```python
from build123d import *

# Parameters (mm, degrees)
F1_DEPTH = 18
F2_R     = 7.5
F3_DEPTH = 25
F4_R     = 1
F5_SIZE  = 1


with BuildPart() as f1:
    # F0 (on Top) → F1 (new body)
    with BuildSketch(Plane.XY):
        with BuildLine():
            Line((-67.585714, 12.773849), (-90.89085, 17.178571))
            ThreePointArc((-90.89085, 17.178571), (-92.5, 0), (-90.89085, -17.178571))
            Line((-90.89085, -17.178571), (-67.585714, -12.773849))
            ThreePointArc((-67.585714, -12.773849), (-57, 0), (-67.585714, 12.773849))
        make_face()
    extrude(amount=F1_DEPTH)

    # F2 (on face) → F3 (join)
    with BuildSketch(Plane.XY.offset(18)):
        with Locations((-70, 0)):
            Circle(F2_R)
    extrude(amount=F3_DEPTH)

    # F4
    f4_edges = [f1.edges().sort_by_distance(p)[0] for p in [
        (-77.5, 0, 18),
        (-79.238282, 14.97621, 18),
    ]]
    fillet(f4_edges, radius=F4_R)

    # F5
    f5_edges = [f1.edges().sort_by_distance(p)[0] for p in [
        (-77.5, 0, 43),
    ]]
    chamfer(f5_edges, length=F5_SIZE)


solid = f1.part
```
Here's how the part is built. I have some questions about the finished solid (model axes, mm). A direction names the side the tool comes from. Coordinates: 2 decimals unless noted, no trailing zeros. Order: outer loops, then holes, each group sorted by start corner. A loop starts at its lowest first (then second) coordinate and runs counter-clockwise, first axis right, second up. Notation, with made-up numbers: (76.5, 20) - (89.5, 20) arc R14 cw to (89.5, 26) - close; hole circle Ø1 at (52.25, 40). An arc over 180 degrees is marked (long way). One line per question, with ' | ' between items.
(1) Suppose I cut it at C-C on z = 4.5. List the corners of the cut face in (x, y) for me, and give its area (3 significant figures).
Report:
outline: (-90.89, -17.18) - (-67.59, -12.77) arc R13 ccw to (-67.59, 12.77) - (-90.89, 17.18) arc R92.5 ccw to start | area: 938 mm2
(2) Suppose I cut it at A-A on y = 0. List the corners of the cut face in (x, z) for me.
Report:
outline: (-92.5, 0) - (-57, 0) - (-57, 17) arc R1 ccw to (-58, 18) - (-61.5, 18) arc R1 cw to (-62.5, 19) - (-62.5, 42) - (-63.5, 43) - (-76.5, 43) - (-77.5, 42) - (-77.5, 19) arc R1 cw to (-78.5, 18) - (-92.5, 18) - close
(3) For faces 1 (the cylindrical face through (-77.493, 0.33, 30.339)), 2 (the cylindrical face through (-79.128, -14.665, 17.699)), which set-ups out of +Z, -Z, +X, -X, +Y, -Y let a thin tool reach every point of the face, with its end or its side?
Report:
face 1: +Z | face 2: +Z, +X, -Y
(4) If I drill on L1, parallel to Z at x = -88, y = 2; L2, parallel to Y at x = -65, z = 38; L3, parallel to X at y = -9.5, z = 9, over which ranges is the centre line in solid material (lowest first)?
Report:
L1: z = 0 to 18 | L2: y = -5.59 to 5.59 | L3: x = -92.01 to -61.13
(5) Will these pins go through, and if not, where does the flat tip stop? pin 1 (1.5 mm diameter, centred on x = -69, z = 31.5, fed in from +Y); pin 2 (1 mm diameter, centred on x = -70, y = 9, fed in from -Z); pin 3 (1 mm diameter, centred on x = -70.5, z = 20, fed in from -Y); pin 4 (1.5 mm diameter, centred on x = -81.5, z = 10, fed in from +Y).
Report:
pin 1: stops at y = 7.5 | pin 2: stops at z = 0 | pin 3: stops at y = -7.5 | pin 4: stops at y = 15.55
(6) Suppose I cut it at B-B on z = 27.5. List the corners of the cut face in (x, y) for me, and give its area (3 significant figures).
Report:
outline: circle Ø15 at (-70, 0) | area: 177 mm2
